Verification items for the finished model (mm, model axes). A direction names the side the tool comes from. Coordinates: 2 decimals unless noted, no trailing zeros. Order: outer loops, then holes, each group sorted by start corner. A loop starts at its lowest first (then second) coordinate and runs counter-clockwise, first axis right, second up. Notation, with made-up numbers: (-33.5, -3.75) -> (10.5, -3.75) arc R9 cw to (10.5, 10.25) -> close; hole circle Ø3 at (5.5, 40). An arc over 180 degrees is marked (long way). Write each question's results on one line, items separated by ' | '. Start each with the question number.
(1) Set-up check for faces 1 (the flat face through (4, 4, -10)), 2 (the flat face through (4, 10, -4)), 3 (the flat face through (4, -10, 4)): record each of +Z, -Z, +X, -X, +Y, -Y from which the full face is reachable in a straight line by a thin tool's end or side.
(2) Thickness scan on probe 1 along Y at (x, z) = (122.5, 9); probe 2 along Z at (x, y) = (-175.5, 0). Record the ranges inside material, lowest first. Write a range as [from, to].
(3) Draft check along Z on faces 4 (the flat face through (4, -4, -10)), 5 (the flat face through (4, -10, -4)). Enter one of: +Z half, -Z half, draft (parallel to the pull), parting line (faces both ways), or undercut.
(4) Cross-section at A-A on x = -213.5. Enter the section's corners in (y, z).
(5) Go/stop test with flat-tipped pins: pin 1 (9 mm diameter, centred on x = 107, z = 1.5, fed in from +Y); pin 2 (2 mm diameter, centred on x = -209, y = -0.5, fed in from -Z); pin 3 (4 mm diameter, centred on x = 98.5, y = -1.5, fed in from +Z); pin 4 (5.5 mm diameter, centred on y = 0, z = 0, fed in from +X). Record where each tip stops, or that it passes through.
```python
from build123d import *

# Parameters (mm, degrees)
F1_DEPTH = 300
F2_R     = 3.4
F3_DEPTH = 600
F4_R     = 3


with BuildPart() as f1:
    # F0 (on Right) → F1 (new body, symmetric)
    with BuildSketch(Plane.YZ):
        Polygon((15, 4), (15, 15), (4, 15), (4, 5), (-4, 5), (-4, 15), (-15, 15), (-15, 4), (-5, 4), (-5, -4), (-15, -4), (-15, -15), (-4, -15), (-4, -5), (4, -5), (4, -15), (15, -15), (15, -4), (5, -4), (5, 4), align=None)
    extrude(amount=F1_DEPTH, both=True)

    # F2 (on face) → F3 (cut)
    with BuildSketch(Plane.YZ.offset(300)):
        Circle(F2_R)
    extrude(amount=-F3_DEPTH, mode=Mode.SUBTRACT)

    # F4
    f4_edges = [f1.edges().sort_by_distance(p)[0] for p in [
        (0, 15, -15),
        (0, 15, 15),
        (0, -15, -15),
        (0, -15, 15),
    ]]
    fillet(f4_edges, radius=F4_R)


solid = f1.part
```
Results are:
1) face 1: -Z, +X, -X | face 2: +X, -X, +Y | face 3: +X, -X, -Y
2) probe 1: y = [-15, -4], [4, 15] | probe 2: z = [-5, -3.4], [3.4, 5]
3) face 4: draft | face 5: undercut
4) outline: (-15, -12) arc R3 ccw to (-12, -15) -> (-4, -15) -> (-4, -5) -> (4, -5) -> (4, -15) -> (12, -15) arc R3 ccw to (15, -12) -> (15, -4) -> (5, -4) -> (5, 4) -> (15, 4) -> (15, 12) arc R3 ccw to (12, 15) -> (4, 15) -> (4, 5) -> (-4, 5) -> (-4, 15) -> (-12, 15) arc R3 ccw to (-15, 12) -> (-15, 4) -> (-5, 4) -> (-5, -4) -> (-15, -4) -> close; hole circle Ø6.8 at (0, 0)
5) pin 1: stops at y = 15 | pin 2: stops at z = -5 | pin 3: stops at z = 5 | pin 4: passes through
